The listing builds one solid part. Answer for the finished solid, in the listing's coordinates (mm). Face numbers are marked on the shaded views. A direction names the side the tool comes from. Coordinates: 2 decimals unless noted, no trailing zeros. Loops run counter-clockwise (first coordinate to the right, second up) from the corner with the lowest first, then second, coordinate; pieces in that order, holes last. Notation, with made-up numbers: (54, 2) - (110, 2) arc R30 ccw to (110, 31) - close; hole circle Ø9 at (42.25, 23). An arc over 180 degrees is marked (long way). Return JSON: item names as keys, results as strings. Group by question number.
1. The mould has two halves that part along X. Classify the marked faces 3, 4 and 5: pulls with the +X half, pulls with the -X half, needs draft (parallel to the pull), parting line crosses it, or undercut.
2. Section A-A (z = 0) is taken. Write down the section's boundary in (x, y), and give its area (3 significant figures).
3. Which of the six approach directions +Z, -Z, +X, -X, +Y, -Y give full straight-line access (tool end or side, diameter ignored) to the marked faces 1 and 2?
4. Each of these flat-tipped pins is pushed along its axis until it touches: P1, Ø2.5, axis at x = -5.5, y = -0.5, coming from the +Z side; P2, Ø4.5, axis at x = 118.5, z = 1, coming from the +Y side; P3, Ø4.5, axis at x = 111.5, z = 1.5, coming from the -Y side. Where does it stop, or does it pass through?
5. Find the intervals of material crossed by line 1 along X through (y, z) = (-4.5, -5); line 2 along X through (y, z) = (-5, 0.25); line 3 along Y through (x, z) = (96, -3.75), in increasing order.
6. Section C-C (x = 68) is taken. Write down the section's boundary in (y, z).
7. Section D-D (x = 105.5) is taken. Write down the section's boundary in (y, z), and give its area (3 significant figures).
```python
from build123d import *

# Parameters (mm, degrees)
SCHNITT_LINEAR_AUSTRAGEN1_DEPTH      = 143.352054199
SCHNITT_LINEAR_AUSTRAGEN1_DEPTH_BACK = 143.352054199
SKIZZE4_W                            = 80.01116069
SKIZZE4_H                            = 4.996766738
SCHNITT_LINEAR_AUSTRAGEN2_DEPTH      = 143.867446828
SCHNITT_LINEAR_AUSTRAGEN2_DEPTH_BACK = 1.9


# Read off the part's stored shape, not the designer's step: M12 Maschinengewinde Bolzen1
with BuildPart() as part:
    # Skizze2 → Rotation1 (revolve)
    with BuildSketch(Plane.XY, mode=Mode.PRIVATE) as rotation1_sk:
        Polygon((-70.992580001, 0), (-70.992580001, 6), (-55.492580001, 6), (-55.492580001, 7), (3.507419999, 7), (3.507419999, 6), (14.507419999, 6), (14.507419999, 7), (92.007419999, 7), (92.007419999, 6), (142.007419999, 6), (142.007419999, 0), align=None)
    revolve(rotation1_sk.sketch.rotate(Axis((-31.289719626, 0, 0), (1, 0, 0)), 90), axis=Axis((-31.289719626, 0, 0), (1, 0, 0)))

    # M12 Maschinengewinde Bolzen1 outline → M12 Maschinengewinde Bolzen1 (revolve, cut)
    with BuildSketch(Plane.YX):
        with BuildLine():
            Line((6, 95.507419999), (5.133974596, 94.007419999))
            ThreePointArc((5.133974596, 94.007419999), (5.034074174, 93.766239044), (5, 93.507419999))
            Line((5, 93.507419999), (5, 93.007419999))
            ThreePointArc((5, 93.007419999), (5.292893219, 92.300313218), (6, 92.007419999))
            Line((6, 92.007419999), (6, 95.507419999))
        make_face()
        Polygon((5.036, 142.007419999), (6, 141.043419999), (6, 142.007419999), align=None)
    revolve(axis=Axis((0, 0, 0), (1, 0, 0)), mode=Mode.SUBTRACT)

    # Skizze4 → Schnitt-Linear austragen1 (cut, two sides: drawn at the far end of the back side and taken through both)
    with BuildSketch(Plane.XY.offset(-SCHNITT_LINEAR_AUSTRAGEN1_DEPTH_BACK)):
        with Locations((132.013000344, 6.498383369)):
            Rectangle(SKIZZE4_W, SKIZZE4_H)
        with Locations((132.013000344, -6.498383369)):
            Rectangle(SKIZZE4_W, SKIZZE4_H)
    extrude(amount=SCHNITT_LINEAR_AUSTRAGEN1_DEPTH + SCHNITT_LINEAR_AUSTRAGEN1_DEPTH_BACK, mode=Mode.SUBTRACT)

    # Skizze5 → Schnitt-Linear austragen2 (cut, two sides: drawn at the far end of the back side and taken through both)
    with BuildSketch(Plane.XY.offset(7).offset(-SCHNITT_LINEAR_AUSTRAGEN2_DEPTH_BACK)):
        with BuildLine():
            Line((-1.492580001, -2.5), (-8.492580001, -2.5))
            ThreePointArc((-8.492580001, -2.5), (-10.992580001, 0), (-8.492580001, 2.5))
            Line((-8.492580001, 2.5), (-1.492580001, 2.5))
            ThreePointArc((-1.492580001, 2.5), (1.007419999, 0), (-1.492580001, -2.5))
        make_face()
    extrude(amount=SCHNITT_LINEAR_AUSTRAGEN2_DEPTH + SCHNITT_LINEAR_AUSTRAGEN2_DEPTH_BACK, mode=Mode.SUBTRACT)


solid = part.part
```
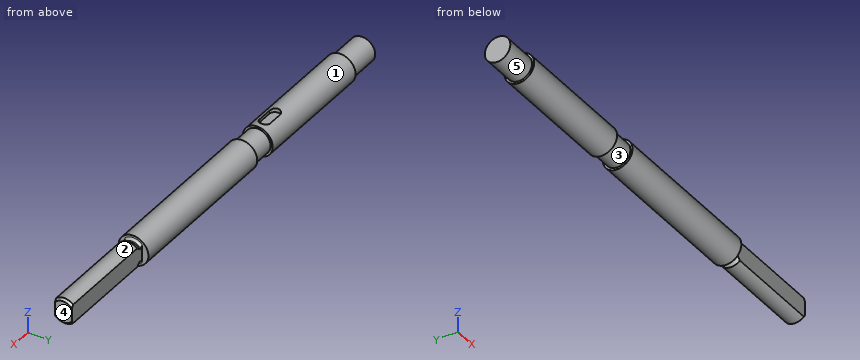
The answers:
{
 "1": {"face 3": "undercut", "face 4": "pulls with the +X half", "face 5": "needs draft"},
 "2": {"outline": "(-70.99, -6) - (-55.49, -6) - (-55.49, -7) - (3.51, -7) - (3.51, -6) - (14.51, -6) - (14.51, -7) - (92.01, -7) - (92.01, -4) - (142.01, -4) - (142.01, 4) - (92.01, 4) - (92.01, 7) - (14.51, 7) - (14.51, 6) - (3.51, 6) - (3.51, 7) - (-55.49, 7) - (-55.49, 6) - (-70.99, 6) - close", "area": "2,630 mm2"},
 "3": {"face 1": "+X, -X", "face 2": "+Z, +X"},
 "4": {"P1": "stops at z = 5.1", "P2": "stops at y = 4", "P3": "stops at y = -4"},
 "5": {"line 1": "x = -55.49 to 3.51, 14.51 to 92.01", "line 2": "x = -70.99 to 92.01", "line 3": "y = -4 to 4"},
 "6": {"outline": "circle Ø14 at (0, 0)"},
 "7": {"outline": "(-4, -4.47) arc R6 ccw to (4, -4.47) - (4, 4.47) arc R6 ccw to (-4, 4.47) - close", "area": "88.3 mm2"}
}
